from build123d import *

# Parameters (mm, degrees)
SKETCH_1_W          = 153
SKETCH_1_H          = 160
EXTRUDE_1_DEPTH     = 3
SKETCH_2_R          = 2.25
CUT_EXTRUDE_1_DEPTH = 5
SKETCH_3_W          = 45
SKETCH_3_H          = 36
CUT_EXTRUDE_2_DEPTH = 5
FILLET_1_R          = 10
CHAMFER_1_SIZE      = 20


with BuildPart() as part:
    # 草图1 → 凸台-拉伸1 (new body)
    with BuildSketch(Plane(origin=(0, 0, 0), x_dir=(1, 0, 0), z_dir=(0, 1, 0))):
        Rectangle(SKETCH_1_W, SKETCH_1_H)
    extrude(amount=EXTRUDE_1_DEPTH)

    # 草图2 → 切除-拉伸1 (cut)
    with BuildSketch(Plane(origin=(0, 3, 0), x_dir=(1, 0, 0), z_dir=(0, 1, 0))):
        with Locations(Location((72.7, 47.5, 0), (0, 0, 270))):
            Circle(SKETCH_2_R)
        with Locations(Location((-72.7, 47.5, 0), (0, 0, 270))):
            Circle(SKETCH_2_R)
        with Locations(Location((72.7, 22.5, 0), (0, 0, 270))):
            Circle(SKETCH_2_R)
        with Locations(Location((-72.7, 22.5, 0), (0, 0, 270))):
            Circle(SKETCH_2_R)
        with Locations(Location((-14, 71.6, 0), (0, 0, 270))):
            Circle(SKETCH_2_R)
        with Locations(Location((14, 71.6, 0), (0, 0, 270))):
            Circle(SKETCH_2_R)
        with Locations(Location((0, 44.1, 0), (0, 0, 270))):
            Circle(SKETCH_2_R)
    extrude(amount=-CUT_EXTRUDE_1_DEPTH, mode=Mode.SUBTRACT)

    # 草图3 → 切除-拉伸2 (cut)
    with BuildSketch(Plane(origin=(0, 3, 0), x_dir=(1, 0, 0), z_dir=(0, 1, 0))):
        with Locations((36, 44.1)):
            Rectangle(SKETCH_3_W, SKETCH_3_H)
        with Locations((-36, 44.1)):
            Rectangle(SKETCH_3_W, SKETCH_3_H)
    extrude(amount=-CUT_EXTRUDE_2_DEPTH, mode=Mode.SUBTRACT)

    # 圆角1
    fillet_1_edges = [part.edges().sort_by_distance(p)[0] for p in [
        (58.5, 1.5, -62.1),
        (58.5, 1.5, -26.1),
        (13.5, 1.5, -26.1),
        (13.5, 1.5, -62.1),
        (-58.5, 1.5, -62.1),
        (-13.5, 1.5, -62.1),
        (-13.5, 1.5, -26.1),
        (-58.5, 1.5, -26.1),
    ]]
    fillet(fillet_1_edges, radius=FILLET_1_R)

    # 倒角1
    chamfer_1_edges = [part.edges().sort_by_distance(p)[0] for p in [
        (-76.5, 1.5, -80),
        (76.5, 1.5, -80),
    ]]
    chamfer(chamfer_1_edges, length=CHAMFER_1_SIZE)


solid = part.part
Build history of the part. All positions in model axes, mm. A direction names the side the tool comes from. Round coordinates to 2 decimals unless told otherwise and drop trailing zeros. Write each loop counter-clockwise with the first axis right and the second up, starting at its lowest first coordinate (ties: lowest second). Pieces come first, ordered by that corner, then holes. Notation, with made-up numbers: (27.5, 63.25) - (35.5, 63.25) arc R12 cw to (35.5, 73.25) - close; hole circle Ø5 at (32.5, 66.25). An arc over 180 degrees is marked (long way). Use CSV: the item, a comma, the result in double quotes.
(1) Band-saw the part on C-C (x = -72.7). Write the cut outline in (y, z).
Response:
outline,"(0, -63.8) - (3, -63.8) - (3, -49.75) - (0, -49.75) - close; (0, -45.25) - (3, -45.25) - (3, -24.75) - (0, -24.75) - close; (0, -20.25) - (3, -20.25) - (3, 80) - (0, 80) - close"
(2) Pin check, flat tip, straight feed: P1, Ø2.5, axis at x = 72.7, z = -22.5, coming from the +Y side. Stop position of the tip, or through.
Response:
P1,"through"
(3) Band-saw the part on B-B (z = -71.6). Write the cut outline in (x, y).
Response:
outline,"(-64.9, 0) - (-16.25, 0) - (-16.25, 3) - (-64.9, 3) - close; (-11.75, 0) - (11.75, 0) - (11.75, 3) - (-11.75, 3) - close; (16.25, 0) - (64.9, 0) - (64.9, 3) - (16.25, 3) - close"
(4) Wall check: line 1 (X direction, y = 0.95, z = -22.5); line 2 (X direction, y = 1.9, z = -35.5); line 3 (X direction, y = 1.15, z = -47.5). Give the ranges that are in metal, low to high.
Response:
line 1,"-76.5 to -74.95, -70.45 to 70.45, 74.95 to 76.5"
line 2,"-76.5 to -58.48, -13.52 to 13.52, 58.48 to 76.5"
line 3,"-76.5 to -74.95, -70.45 to -58.5, -13.5 to 13.5, 58.5 to 70.45, 74.95 to 76.5"
(5) 3-axis set-ups, long thin cutter, end or side, ignore diameter. For faces 1 (the cylindrical face through (16.51, 1.48, -28.95)), 2 (the flat face through (66.6, 1.5, -69.9)): which of +Z, -Z, +X, -X, +Y, -Y reach the whole face in a straight line?
Response:
face 1,"+Y, -Y"
face 2,"-Z, +X, +Y, -Y"
(6) Band-saw the part on A-A (x = 0). Write the cut outline in (y, z), plus the area to 4 significant figures.
Response:
outline,"(0, -80) - (3, -80) - (3, -46.35) - (0, -46.35) - close; (0, -41.85) - (3, -41.85) - (3, 80) - (0, 80) - close"
area,"466.5 mm²"
(7) Mould opens along Z. For faces 3 (the cylindrical face through (-72.601, 1.521, -49.748)), 4 (the flat face through (-66.4, 1.5, -70.1)), 5 (the flat face through (-1, 3, 17)) say: pulls with the +Z half, pulls with the -Z half, needs draft (parallel to the pull), parting line crosses it, or undercut.
Response:
face 3,"undercut"
face 4,"pulls with the -Z half"
face 5,"needs draft"
(8) Band-saw the part on D-D (y = 1.45). Give the number of separate pieces and of enclosed holes in the cut face, plus the area to 3 significant figures.
Response:
separate pieces,"1"
enclosed holes,"9"
area,"20,900 mm²"
